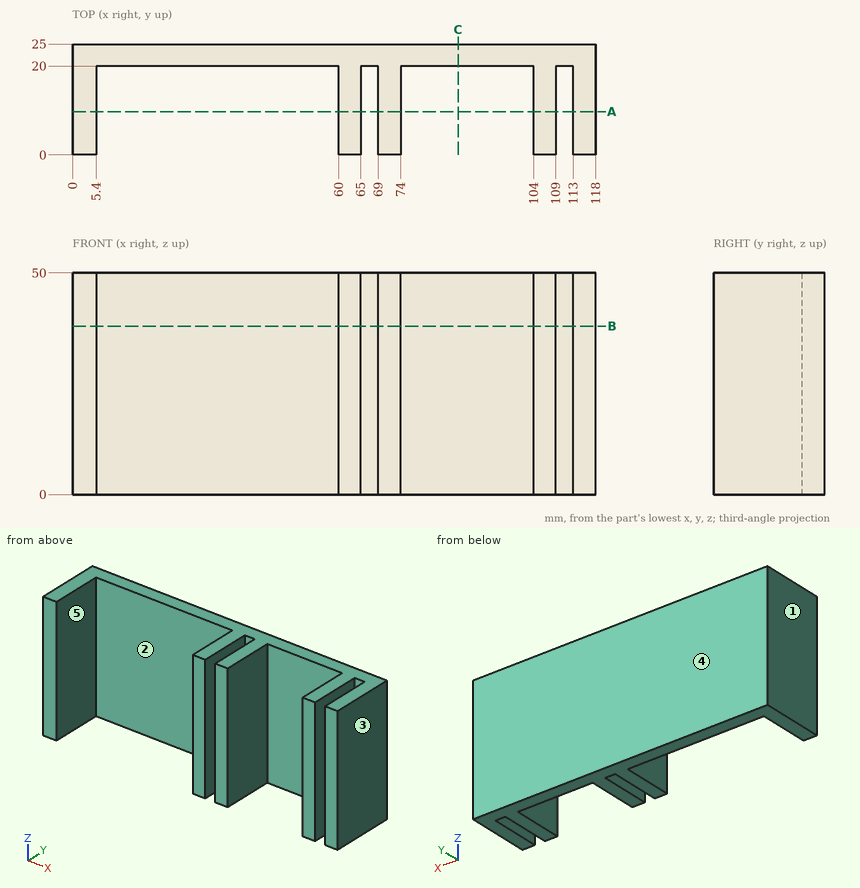
Geometry: see drawing. Coordinates: mm, zero at the bounding-box minimum. A direction names the side the tool comes from. Round coordinates to 2 decimals unless told otherwise and drop trailing zeros. Loops run counter-clockwise (first coordinate to the right, second up) from the corner with the lowest first, then second, coordinate; pieces in that order, holes last. Notation, with made-up numbers: M 77.25,-0.5 L 82.25,-0.5 A29 ccw 82.25,21.5 Z; hole C 28,75.5 d7. An arc over 180 degrees is marked long. Use a Markdown table: item, result. Add a question column.
1. Line query: line 1 (X direction, y = 17.5, z = 6); line 2 (Y direction, x = 24.5, z = 46). Output: solid intervals per line, ascending.
2. Section query A-A on y = 9.75. Return the cut outline in (x, z), then the cut area to 3 significant figures.
3. Contact query for a flat-ended pin moving along its axis: P1, Ø2, axis at x = 66.5, z = 36, coming from the -Y side. Output: stop coordinate, or through.
4. Section query B-B on z = 38. Return the cut outline in (x, y), then the cut area to 3 significant figures.
5. Section query C-C on x = 87. Return the cut outline in (y, z), then the cut area to 3 significant figures.
6. Reachability of the marked faces 1 and 2 from +Z, -Z, +X, -X, +Y, -Y: full face, straight path, thin tool, end or side. Return the list, or none.
7. Mould query, pull axis X, two halves, no side actions, for the marked faces 3, 4 and 5. Classes: pulls with the +X half, pulls with the -X half, needs draft (parallel to the pull), parting line crosses it, or undercut.
Reported:
| question | item | result |
|---|---|---|
| 1 | line 1 | x = 0 to 5.4, 60 to 65, 69 to 74, 104 to 109, 113 to 118 |
| 1 | line 2 | y = 20 to 25 |
| 2 | outline | M 0,0 L 5.4,0 L 5.4,50 L 0,50 Z; M 60,0 L 65,0 L 65,50 L 60,50 Z; M 69,0 L 74,0 L 74,50 L 69,50 Z; M 104,0 L 109,0 L 109,50 L 104,50 Z; M 113,0 L 118,0 L 118,50 L 113,50 Z |
| 2 | area | 1,270 mm² |
| 3 | P1 | stops at y = 20 |
| 4 | outline | M 0,0 L 5.4,0 L 5.4,20 L 60,20 L 60,0 L 65,0 L 65,20 L 69,20 L 69,0 L 74,0 L 74,20 L 104,20 L 104,0 L 109,0 L 109,20 L 113,20 L 113,0 L 118,0 L 118,25 L 0,25 Z |
| 4 | area | 1,100 mm² |
| 5 | outline | M 20,0 L 25,0 L 25,50 L 20,50 Z |
| 5 | area | 250 mm² |
| 6 | face 1 | +Z, -Z, -X, +Y, -Y |
| 6 | face 2 | +Z, -Z, -Y |
| 7 | face 3 | pulls with the +X half |
| 7 | face 4 | needs draft |
| 7 | face 5 | undercut |
